from build123d import *

# Parameters (mm, degrees)
CROQUIS1_W                 = 100
CROQUIS1_H                 = 70
SALIENTE_EXTRUIR1_DEPTH    = 10
CORTAR_EXTRUIR1_DEPTH      = 6.5
CROQUIS5_R                 = 4
CORTAR_EXTRUIR2_DEPTH      = 10
CHAFL_N1_SIZE              = 1.5
CHAFL_N1_OF_SIMETR_A1_SIZE = 1.5
REDONDEO4_R                = 20
REDONDEO5_R                = 20
REDONDEO6_R                = 20
REDONDEO7_R                = 20
CORTAR_EXTRUIR3_DEPTH      = 10


with BuildPart() as part:
    # Croquis1 → Saliente-Extruir1 (new body)
    with BuildSketch(Plane(origin=(0, 0, 0), x_dir=(1, 0, 0), z_dir=(0, 1, 0))):
        with Locations((50, 35)):
            Rectangle(CROQUIS1_W, CROQUIS1_H)
    extrude(amount=SALIENTE_EXTRUIR1_DEPTH)

    # Croquis2 → Cortar-Extruir1 (cut)
    with BuildSketch(Plane(origin=(0, 10, 0), x_dir=(1, 0, 0), z_dir=(0, 1, 0))):
        Polygon((12.5, 42.25), (6.221315823, 38.625), (6.221315823, 31.375), (12.5, 27.75), (18.778684177, 31.375), (18.778684177, 38.625), align=None)
    cortar_extruir1 = extrude(amount=-CORTAR_EXTRUIR1_DEPTH, mode=Mode.SUBTRACT)

    # Croquis5 → Cortar-Extruir2 (cut)
    with BuildSketch(Plane(origin=(0, 10, 0), x_dir=(1, 0, 0), z_dir=(0, 1, 0))):
        with Locations(Location((12.5, 35, 0), (0, 0, 270))):
            Circle(CROQUIS5_R)
    cortar_extruir2 = extrude(amount=-CORTAR_EXTRUIR2_DEPTH, mode=Mode.SUBTRACT)

    # Chaflán1
    chafl_n1_edges = [part.edges().sort_by_distance(p)[0] for p in [
        (15.639342089, 10, -40.4375),
        (9.360657911, 10, -40.4375),
        (6.221315823, 10, -35),
        (9.360657911, 10, -29.5625),
        (15.639342089, 10, -29.5625),
        (18.778684177, 10, -35),
    ]]
    chamfer(chafl_n1_edges, length=CHAFL_N1_SIZE)

    # Simetría1: Cortar-Extruir1, Cortar-Extruir2 across plane
    add(cortar_extruir1.mirror(Plane.ZY.offset(-50)), mode=Mode.SUBTRACT)
    add(cortar_extruir2.mirror(Plane.ZY.offset(-50)), mode=Mode.SUBTRACT)

    # Chaflán1 of Simetría1
    chafl_n1_of_simetr_a1_edges = [part.edges().sort_by_distance(p)[0] for p in [
        (84.360657911, 10, -40.4375),
        (90.639342089, 10, -40.4375),
        (93.778684177, 10, -35),
        (90.639342089, 10, -29.5625),
        (84.360657911, 10, -29.5625),
        (81.221315823, 10, -35),
    ]]
    chamfer(chafl_n1_of_simetr_a1_edges, length=CHAFL_N1_OF_SIMETR_A1_SIZE)

    # Redondeo4
    redondeo4_edges = [part.edges().sort_by_distance(p)[0] for p in [
        (100, 5, -70),
    ]]
    fillet(redondeo4_edges, radius=REDONDEO4_R)

    # Redondeo5
    redondeo5_edges = [part.edges().sort_by_distance(p)[0] for p in [
        (100, 5, 0),
    ]]
    fillet(redondeo5_edges, radius=REDONDEO5_R)

    # Redondeo6
    redondeo6_edges = [part.edges().sort_by_distance(p)[0] for p in [
        (0, 5, 0),
    ]]
    fillet(redondeo6_edges, radius=REDONDEO6_R)

    # Redondeo7
    redondeo7_edges = [part.edges().sort_by_distance(p)[0] for p in [
        (0, 5, -70),
    ]]
    fillet(redondeo7_edges, radius=REDONDEO7_R)

    # Croquis7 → Cortar-Extruir3 (cut)
    with BuildSketch(Plane(origin=(0, 10, 0), x_dir=(1, 0, 0), z_dir=(0, 1, 0))):
        with BuildLine():
            Line((30, 13), (70, 13))
            ThreePointArc((70, 13), (72.5, 10.5), (70, 8))
            Line((70, 8), (30, 8))
            ThreePointArc((30, 8), (27.5, 10.5), (30, 13))
        make_face()
        with BuildLine():
            Line((30, 18), (70, 18))
            ThreePointArc((70, 18), (72.5, 20.5), (70, 23))
            Line((70, 23), (30, 23))
            ThreePointArc((30, 23), (27.5, 20.5), (30, 18))
        make_face()
        with BuildLine():
            Line((30, 28), (70, 28))
            ThreePointArc((70, 28), (72.5, 30.5), (70, 33))
            Line((70, 33), (30, 33))
            ThreePointArc((30, 33), (27.5, 30.5), (30, 28))
        make_face()
        with BuildLine():
            Line((30, 38), (70, 38))
            ThreePointArc((70, 38), (72.5, 40.5), (70, 43))
            Line((70, 43), (30, 43))
            ThreePointArc((30, 43), (27.5, 40.5), (30, 38))
        make_face()
        with BuildLine():
            Line((30, 48), (70, 48))
            ThreePointArc((70, 48), (72.5, 50.5), (70, 53))
            Line((70, 53), (30, 53))
            ThreePointArc((30, 53), (27.5, 50.5), (30, 48))
        make_face()
        with BuildLine():
            Line((30, 58), (70, 58))
            ThreePointArc((70, 58), (72.5, 60.5), (70, 63))
            Line((70, 63), (30, 63))
            ThreePointArc((30, 63), (27.5, 60.5), (30, 58))
        make_face()
    extrude(amount=-CORTAR_EXTRUIR3_DEPTH, mode=Mode.SUBTRACT)


solid = part.part
Part model, mm, in its own coordinate system. A direction names the side the tool comes from. Coordinates: 2 decimals unless noted, no trailing zeros. Order: outer loops, then holes, each group sorted by start corner. A loop starts at its lowest first (then second) coordinate and runs counter-clockwise, first axis right, second up. Notation, with made-up numbers: (29.5, 15) - (63.5, 15) arc R14 cw to (63.5, 19) - close; hole circle Ø4 at (65, 78.25). An arc over 180 degrees is marked (long way). Use CSV: the item, a comma, the result in double quotes.
Item 1: 3-axis set-ups, long thin cutter, end or side, ignore diameter. For faces 1 (the face through (9.05, 9.24, -41.11)), 2 (the face through (100, 5, -35)), 3 (the face through (27.5, 5.1, -10.4)): which of +Z, -Z, +X, -X, +Y, -Y reach the whole face in a straight line?
Solved:
face 1,"+Y"
face 2,"+Z, -Z, +X, +Y, -Y"
face 3,"+Y, -Y"
Item 2: Saw through at A-A on x = 68.5. Give the cut face in (y, z), and give its area (3 significant figures).
Solved:
outline,"(0, -70) - (10, -70) - (10, -63) - (0, -63) - close; (0, -58) - (10, -58) - (10, -53) - (0, -53) - close; (0, -48) - (10, -48) - (10, -43) - (0, -43) - close; (0, -38) - (10, -38) - (10, -33) - (0, -33) - close; (0, -28) - (10, -28) - (10, -23) - (0, -23) - close; (0, -18) - (10, -18) - (10, -13) - (0, -13) - close; (0, -8) - (10, -8) - (10, 0) - (0, 0) - close"
area,"400 mm²"
Item 3: Probe probe 1 along X at (y, z) = (1.55, -35); probe 2 along X at (y, z) = (5.5, -20.5); probe 3 along X at (y, z) = (4.5, -32). List the from-to ranges inside material, lowest first.
Solved:
probe 1,"x = 0 to 8.5, 16.5 to 83.5, 91.5 to 100"
probe 2,"x = 0 to 27.5, 72.5 to 100"
probe 3,"x = 0 to 6.22, 18.78 to 28, 72 to 81.22, 93.78 to 100"
Item 4: Saw through at C-C on y = 1.25. Give the number of separate pieces and of enclosed holes in the cut face, and give its area (3 significant figures).
Solved:
separate pieces,"1"
enclosed holes,"8"
area,"5,240 mm²"
Item 5: Saw through at B-B on z = -35. Give the cut face in (x, y), and give its area (3 significant figures).
Solved:
outline,"(0, 0) - (8.5, 0) - (8.5, 3.5) - (6.22, 3.5) - (6.22, 8.5) - (4.72, 10) - (0, 10) - close; (16.5, 0) - (83.5, 0) - (83.5, 3.5) - (81.22, 3.5) - (81.22, 8.5) - (79.72, 10) - (20.28, 10) - (18.78, 8.5) - (18.78, 3.5) - (16.5, 3.5) - close; (91.5, 0) - (100, 0) - (100, 10) - (95.28, 10) - (93.78, 8.5) - (93.78, 3.5) - (91.5, 3.5) - close"
area,"776 mm²"
Item 6: Drop flat-ended pins along their axis: P1, Ø4, axis at x = 84.5, z = -39, coming from the +Y side; P2, Ø10.5, axis at x = 12.5, z = -35, coming from the +Y side; P3, Ø6, axis at y = 1.5, z = -11, coming from the -X side. Give the stop position or say it passes through.
Solved:
P1,"stops at y = 9.19"
P2,"stops at y = 3.5"
P3,"stops at x = 0.92"
Item 7: Mould opens along X. For faces 4 (the face through (84.05, 9.24, -28.89)), 5 (the face through (50, 5, -70)), 6 (the face through (94.297, 5.07, -6.014)), 7 (the face through (50, 5, -58)) say: +X half, -X half, draft (parallel to the pull), parting line (faces both ways), or undercut.
Solved:
face 4,"undercut"
face 5,"draft"
face 6,"+X half"
face 7,"undercut"
Item 8: Saw through at D-D on z = -60.5. Give the cut face in (x, y).
Solved:
outline,"(2.98, 0) - (27.5, 0) - (27.5, 10) - (2.98, 10) - close; (72.5, 0) - (97.02, 0) - (97.02, 10) - (72.5, 10) - close"
